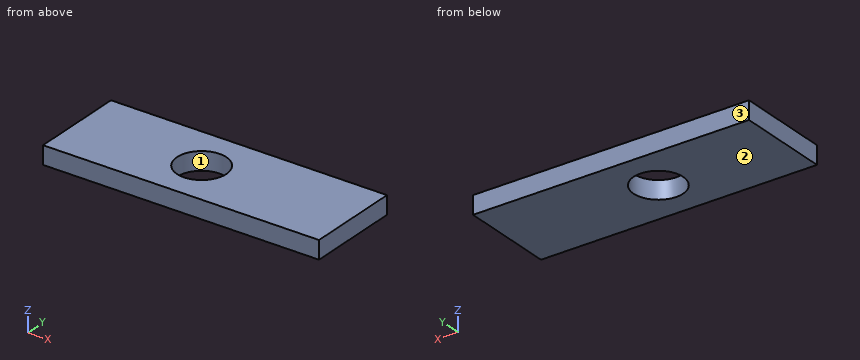
Autodesk Inventor part; units mm, degrees
ref_plane "YZ Plane" through (0, 0, 0) normal (1, 0, 0) x (0, 1, 0)
ref_plane "XZ Plane" through (0, 0, 0) normal (0, 1, 0) x (-1, 0, 0)
ref_plane "XY Plane" through (0, 0, 0) normal (0, 0, 1) x (1, 0, 0)
sketch "Skizze1" plane through (0, 0, 0) normal (0, 0, 1) x (1, 0, 0)
  line L0 (0, 0) -> (24.3, 0)
  line L1 (24.3, 0) -> (24.3, -8.3)
  line L2 (24.3, -8.3) -> (0, -8.3)
  line L3 (0, -8.3) -> (0, 0)
  circle A0 centre (10.975, -4.15) radius 2.175
  dimension "d0" = 8.3
  dimension "d1" = 24.3
  dimension "d2" = 4.15
  dimension "d3" = 4.15
  dimension "d4" = 4.35
  dimension "d5" = 13.325
extrude "Extrusion1" add sketch "Skizze1" along normal blind 1.6
equation "\"d2\" = d3"
properties part number "Grundplatte" material "PBT-Kunststoff"
Read the model definition and answer for the solid it produces. Units are mm, in the model's axes. Face numbers are marked on the shaded views. Round coordinates to 2 decimals unless told otherwise and drop trailing zeros. Order: outer loops, then holes, each group sorted by start corner. A loop starts at its lowest first (then second) coordinate and runs counter-clockwise, first axis right, second up.
1) The mould has two halves that part along Y. Classify the marked faces 1, 2 and 3: released by +Y, released by -Y, zero draft, split by the parting line, or undercut.
2) The part is cut by section B-B on x = 12.75. Write down the section's boundary in (y, z).
3) The part is cut by section A-A on y = -4.15. Write down the section's boundary in (x, z).
4) Straight lines are drawn through the part: L1, parallel to X at y = -5.25, z = 0.8; L2, parallel to X at y = -3.25, z = 0.85; L3, parallel to Y at x = 11.5, z = 0.7. For each, find the intervals that lie inside material, in ascending order.
5) A flat-ended cylindrical pin translates along its axis: pin 1 (3.5 mm diameter, centred on x = 10.975, y = -4.15, fed in from -Z). Find the tip coordinate at first contact, or state that the pin passes through.
6) The part is cut by section C-C on z = 0.95. Write down the section's boundary in (x, y) (3 decimals).
Resolved:
1. face 1: undercut
1. face 2: zero draft
1. face 3: released by +Y
2. outline: (-8.3, 0) - (-5.41, 0) - (-5.41, 1.6) - (-8.3, 1.6) - close; (-2.89, 0) - (0, 0) - (0, 1.6) - (-2.89, 1.6) - close
3. outline: (0, 0) - (8.8, 0) - (8.8, 1.6) - (0, 1.6) - close; (13.15, 0) - (24.3, 0) - (24.3, 1.6) - (13.15, 1.6) - close
4. L1: x = 0 to 9.1, 12.85 to 24.3
4. L2: x = 0 to 8.99, 12.96 to 24.3
4. L3: y = -8.3 to -6.26, -2.04 to 0
5. pin 1: passes through
6. outline: (0, -8.3) - (24.3, -8.3) - (24.3, 0) - (0, 0) - close; hole circle Ø4.35 at (10.975, -4.15)
